```python
from build123d import *

# Parameters (mm, degrees)
RETAINER_FEATURE_1_PROFILE_R  = 3.8
RETAINER_FEATURE_1_DEPTH      = 5.02
RETAINER_FEATURE_2_PROFILE_R  = 6.2
RETAINER_FEATURE_2_DEPTH      = 2.5
RETAINER_FEATURE_5_DEPTH      = 2.5
RETAINER_FEATURE_8_DEPTH      = 2.5
RETAINER_FEATURE_12_DEPTH     = 2.5
RETAINER_FEATURE_13_PROFILE_R = 7.2
RETAINER_FEATURE_13_DEPTH     = 2.5
RETAINER_FEATURE_14_PROFILE_R = 5.5
RETAINER_FEATURE_14_DEPTH     = 2.7
RETAINER_FEATURE_15_PROFILE_R = 1.1
RETAINER_FEATURE_15_DEPTH     = 3.75
RETAINER_FEATURE_16_PROFILE_R = 2.1
RETAINER_FEATURE_16_DEPTH     = 1.45
RETAINER_FEATURE_17_PROFILE_R = 1.1
RETAINER_FEATURE_17_DEPTH     = 3.75
RETAINER_FEATURE_18_PROFILE_R = 2.1
RETAINER_FEATURE_18_DEPTH     = 1.45


with BuildPart() as part:
    # Retainer Feature 1 profile → Retainer Feature 1 (new body)
    with BuildSketch(Plane(origin=(0, -101, 0), x_dir=(-1, 0, 0), z_dir=(0, -1, 0))):
        with Locations(Location((56.291651246, -30, 0), (0, 0, 90))):
            Circle(RETAINER_FEATURE_1_PROFILE_R)
    extrude(amount=RETAINER_FEATURE_1_DEPTH)

    # Retainer Feature 2 profile → Retainer Feature 2 (add)
    with BuildSketch(Plane(origin=(0, -106, 0), x_dir=(-1, 0, 0), z_dir=(0, -1, 0))):
        with Locations(Location((56.291651246, -30, 0), (0, 0, 90))):
            Circle(RETAINER_FEATURE_2_PROFILE_R)
    extrude(amount=RETAINER_FEATURE_2_DEPTH)

    # Middle Right Floating Compression Ball R → Retainer Feature 5 (add)
    with BuildSketch(Plane(origin=(0, -106, 0), x_dir=(-1, 0, 0), z_dir=(0, -1, 0))):
        Polygon((44.791651246, -30), (46.291651246, -32.598076211), (49.291651246, -32.598076211), (50.791651246, -30), (49.291651246, -27.401923789), (46.291651246, -27.401923789), align=None)
    extrude(amount=RETAINER_FEATURE_5_DEPTH)

    # Middle Right Floating Compression Ba 2 → Retainer Feature 8 (add)
    with BuildSketch(Plane(origin=(0, -106, 0), x_dir=(-1, 0, 0), z_dir=(0, -1, 0))):
        Polygon((61.791651246, -30), (63.291651246, -32.598076211), (66.291651246, -32.598076211), (67.791651246, -30), (66.291651246, -27.401923789), (63.291651246, -27.401923789), align=None)
    extrude(amount=RETAINER_FEATURE_8_DEPTH)

    # Retainer Feature 9 profile → Retainer Feature 9 (revolve, cut)
    with BuildSketch(Plane(origin=(0, -101, 0), x_dir=(-1, 0, 0), z_dir=(0, -1, 0))):
        with BuildLine():
            Line((56.291651246, -33.15), (56.291651246, -26.85))
            ThreePointArc((56.291651246, -26.85), (53.141651246, -30), (56.291651246, -33.15))
        make_face()
    revolve(axis=Axis((-56.291651246, -101, 20), (0, 0, 1)), mode=Mode.SUBTRACT)

    # Middle Right Floating Compression Ba 3 → Retainer Feature 12 (add)
    with BuildSketch(Plane(origin=(0, -106, 0), x_dir=(-1, 0, 0), z_dir=(0, -1, 0))):
        Polygon((56.095916768, -32.993607859), (74.095916768, -34.170522395), (74.487385724, -28.183306677), (56.487385724, -27.006392141), align=None)
    extrude(amount=RETAINER_FEATURE_12_DEPTH)

    # Retainer Feature 13 profile → Retainer Feature 13 (add)
    with BuildSketch(Plane(origin=(0, -106, 0), x_dir=(-1, 0, 0), z_dir=(0, -1, 0))):
        with Locations((74.291651246, -31.176914536)):
            Circle(RETAINER_FEATURE_13_PROFILE_R)
    extrude(amount=RETAINER_FEATURE_13_DEPTH)

    # Retainer Feature 14 profile → Retainer Feature 14 (cut)
    with BuildSketch(Plane(origin=(0, -105.9, 0), x_dir=(-1, 0, 0), z_dir=(0, -1, 0))):
        with Locations(Location((74.291651246, -31.176914536, 0), (0, 0, 270))):
            Circle(RETAINER_FEATURE_14_PROFILE_R)
    extrude(amount=RETAINER_FEATURE_14_DEPTH, mode=Mode.SUBTRACT)

    # Retainer Feature 15 profile → Retainer Feature 15 (cut)
    with BuildSketch(Plane(origin=(0, -105, 0), x_dir=(-1, 0, 0), z_dir=(0, -1, 0))):
        with Locations(Location((47.791651246, -30, 0), (0, 0, 90))):
            Circle(RETAINER_FEATURE_15_PROFILE_R)
    extrude(amount=RETAINER_FEATURE_15_DEPTH, mode=Mode.SUBTRACT)

    # Retainer Feature 16 profile → Retainer Feature 16 (cut)
    with BuildSketch(Plane(origin=(0, -107.3, 0), x_dir=(-1, 0, 0), z_dir=(0, -1, 0))):
        with Locations(Location((47.791651246, -30, 0), (0, 0, 90))):
            Circle(RETAINER_FEATURE_16_PROFILE_R)
    extrude(amount=RETAINER_FEATURE_16_DEPTH, mode=Mode.SUBTRACT)

    # Retainer Feature 17 profile → Retainer Feature 17 (cut)
    with BuildSketch(Plane(origin=(0, -105, 0), x_dir=(-1, 0, 0), z_dir=(0, -1, 0))):
        with Locations(Location((64.791651246, -30, 0), (0, 0, 90))):
            Circle(RETAINER_FEATURE_17_PROFILE_R)
    extrude(amount=RETAINER_FEATURE_17_DEPTH, mode=Mode.SUBTRACT)

    # Retainer Feature 18 profile → Retainer Feature 18 (cut)
    with BuildSketch(Plane(origin=(0, -107.3, 0), x_dir=(-1, 0, 0), z_dir=(0, -1, 0))):
        with Locations(Location((64.791651246, -30, 0), (0, 0, 90))):
            Circle(RETAINER_FEATURE_18_PROFILE_R)
    extrude(amount=RETAINER_FEATURE_18_DEPTH, mode=Mode.SUBTRACT)

    # Articulation Throat Sketch → Articulation Throat (revolve, cut)
    with BuildSketch(Plane(origin=(-75.19414337, -14.119516346, 20.509419779), x_dir=(-0.2544785459472912, -0.04778449262394895, -0.9658971539026421), z_dir=(0.9493062747008634, 0.17825517869277502, -0.2589260282064664))):
        Polygon((-9.825663304, -88.876600419), (-8.475389129, -90.738524062), (14.088996194, -82.675837476), (8.793573125, -75.373858667), align=None)
    revolve(axis=Axis((-53.148124615, -106.383086561, 37.819246728), (-0.3143526631246646, 0.5383086561091633, -0.781924672807028)), mode=Mode.SUBTRACT)


solid = part.part
```
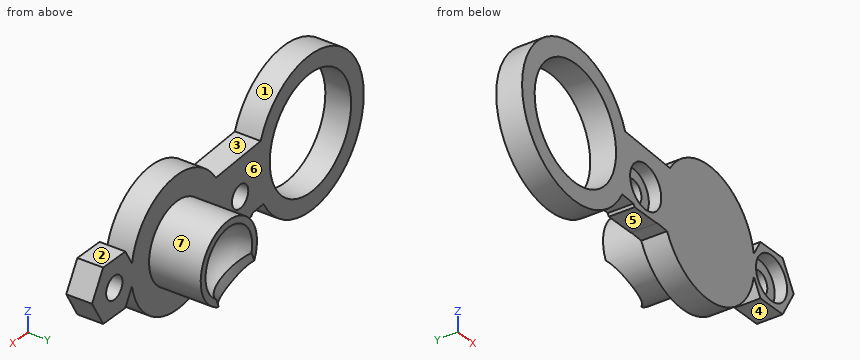
Source: CAD feature listing. Evaluate the final solid. Frame: model axes, mm. Face numbers are marked on the shaded views. A direction names the side the tool comes from. Give positions to 0.01 mm unless a question says otherwise; leave off trailing zeros. Loops run counter-clockwise (first coordinate to the right, second up) from the corner with the lowest first, then second, coordinate; pieces in that order, holes last. Notation, with made-up numbers: (45.25, 33) -> (56.25, 33) arc R17 ccw to (56.25, 53) -> close; hole circle Ø6 at (-34.5, -23.5). An arc over 180 degrees is marked (long way). Use a Markdown table: item, result. Add a question column.
(1) Ray query, line 1 (Z direction, x = -74, y = -107.5); line 2 (X direction, y = -107.75, z = 35.25); line 3 (Y direction, x = -79.5, z = 29). Return the intervals inside material, ascending.
(2) Section query A-A (z = 35.25). Output: boundary loops of the cut face in (x, y), then the cut area to 3 significant figures.
(3) First-contact query: pin 1 Ø2 at (x, y) = (-75.5, -107) entering from -Z; pin 2 Ø1.3 at (x, z) = (-48, 29.5) entering from -Y; pin 3 Ø2 at (x, y) = (-65, -108) entering from -Z. Flat tips, straight axial feed; report the tip coordinate or a pass-through.
(4) Section query C-C (y = -103.25). Output: boundary loops of the cut face in (x, z), then the cut area to 3 significant figures.
(5) Pull-direction query (X, two-part tool) for the marked faces 5, 6 and 7; classes: +X half, -X half, draft (parallel to the pull), parting line (faces both ways), or undercut.
(6) Access query for the marked faces 1, 2, 3 and 4. Directions: +Z, -Z, +X, -X, +Y, -Y. A direction counts if a zero-diameter tool reaches every point of the face in a straight line with its end or side. Return the directions, or none.
(7) Section query B-B (y = -106.5). Output: boundary loops of the cut face in (x, z).
Checked values:
| question | item | result |
|---|---|---|
| 1 | line 1 | 23.98 to 25.68, 36.67 to 38.37 |
| 1 | line 2 | -80.23 to -77.99, -70.6 to -68.35, -59.59 to -52.99 |
| 1 | line 3 | -108.5 to -106 |
| 2 | outline | (-80.23, -108.5) -> (-77.99, -108.5) -> (-77.99, -106) -> (-80.23, -106) -> close; (-70.6, -108.5) -> (-68.35, -108.5) -> (-68.35, -106) -> (-70.6, -106) -> close; (-59.59, -108.5) -> (-52.99, -108.5) -> (-52.99, -106) -> (-59.59, -106) -> close |
| 2 | area | 27.7 mm^2 |
| 3 | pin 1 | z = 23.98 |
| 3 | pin 2 | y = -107.3 |
| 3 | pin 3 | z = 27.4 |
| 4 | outline | circle Ø7.6 at (-56.29, 30); hole circle Ø4.41 at (-56.29, 30) |
| 4 | area | 30.1 mm^2 |
| 5 | face 5 | undercut |
| 5 | face 6 | draft |
| 5 | face 7 | parting line |
| 6 | face 1 | +Y, -Y |
| 6 | face 2 | +Z, +X, +Y, -Y |
| 6 | face 3 | +Z, +Y, -Y |
| 6 | face 4 | -Z, +X, +Y, -Y |
| 7 | outline | (-67.96, 27.76) -> (-66.44, 27.66) -> (-66.29, 27.4) -> (-63.29, 27.4) -> (-63.26, 27.45) -> (-61.9, 27.36) arc R6.2 ccw to (-50.18, 28.94) -> (-49.29, 27.4) -> (-46.29, 27.4) -> (-44.79, 30) -> (-46.29, 32.6) -> (-49.29, 32.6) -> (-50.18, 31.06) arc R6.2 ccw to (-61.51, 33.35) -> (-67.56, 33.74) arc R7.2 ccw (long way) to start; hole circle Ø11 at (-74.29, 31.18); hole circle Ø2.2 at (-64.79, 30); hole circle Ø2.2 at (-47.79, 30) |
